Here's the drawing with two shaded views (mm, measured from the low corner). I have some questions. Coordinates: 2 decimals unless noted, no trailing zeros. Order: outer loops, then holes, each group sorted by start corner. A loop starts at its lowest first (then second) coordinate and runs counter-clockwise, first axis right, second up. Notation, with made-up numbers: (47, -12) - (91, -12) arc R15 ccw to (91, 11) - close; hole circle Ø5 at (57, -27). An arc over 180 degrees is marked (long way). Answer as CSV lines item,"result". Start each with the question number.
1. I want a section at C-C, the plane z = 3.55. List the corners of the cut face in (x, y) for me, and give its area (3 significant figures).
2. I want a section at A-A, the plane y = 6. List the corners of the cut face in (x, z) for me.
3. I want a section at B-B, the plane x = 7.5. List the corners of the cut face in (y, z) for me, and give its area (3 significant figures).
4. I need wall thicknesses on probe 1 along Y at (x, z) = (7.5, 2.95); probe 2 along X at (y, z) = (39, 3.85); probe 3 along Y at (x, z) = (0.75, 3). Which ranges of each line are inside material? Lowest first, please.
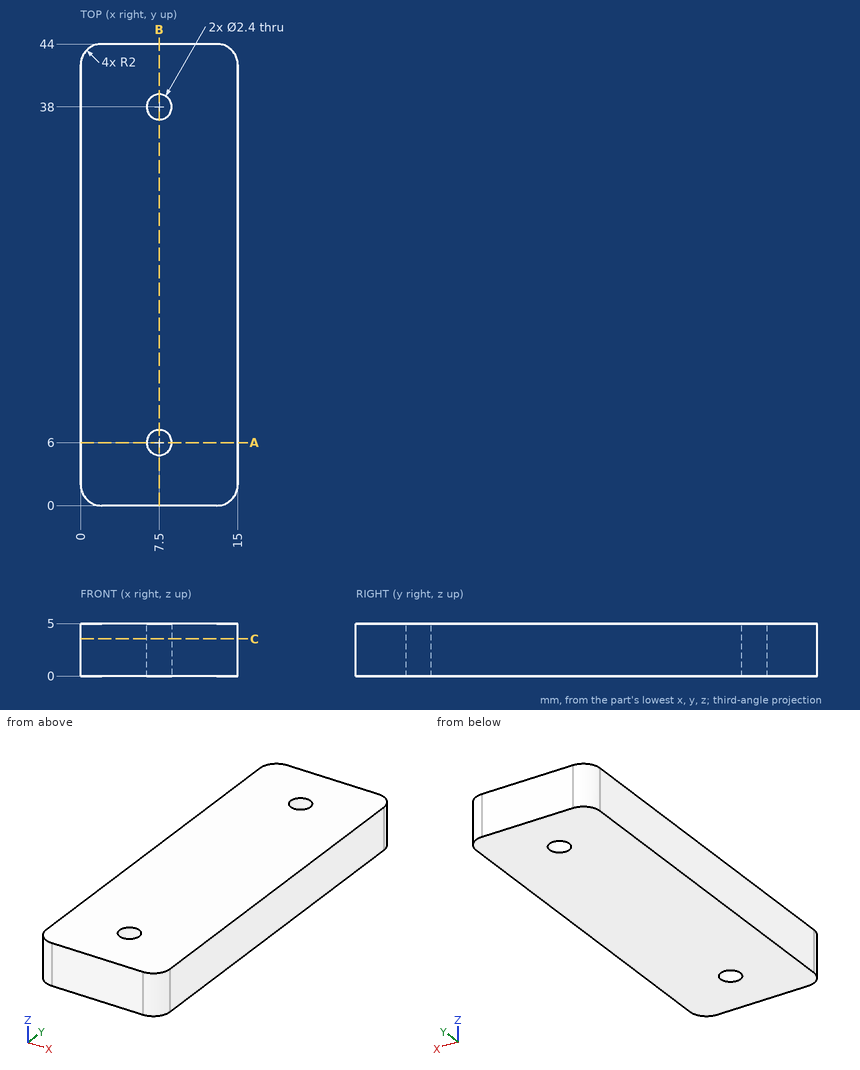
Solved:
1,outline,"(0, 2) arc R2 ccw to (2, 0) - (13, 0) arc R2 ccw to (15, 2) - (15, 42) arc R2 ccw to (13, 44) - (2, 44) arc R2 ccw to (0, 42) - close; hole circle Ø2.4 at (7.5, 6); hole circle Ø2.4 at (7.5, 38)"
1,area,"648 mm2"
2,outline,"(0, 0) - (6.3, 0) - (6.3, 5) - (0, 5) - close; (8.7, 0) - (15, 0) - (15, 5) - (8.7, 5) - close"
3,outline,"(0, 0) - (4.8, 0) - (4.8, 5) - (0, 5) - close; (7.2, 0) - (36.8, 0) - (36.8, 5) - (7.2, 5) - close; (39.2, 0) - (44, 0) - (44, 5) - (39.2, 5) - close"
3,area,"196 mm2"
4,probe 1,"y = 0 to 4.8, 7.2 to 36.8, 39.2 to 44"
4,probe 2,"x = 0 to 6.84, 8.16 to 15"
4,probe 3,"y = 0.44 to 43.56"
